Source: three-view drawing plus pictorial views. Frame: mm from the lowest corner of the part. A direction names the side the tool comes from. Give positions to 0.01 mm unless a question says otherwise; leave off trailing zeros. Order: outer loops, then holes, each group sorted by start corner. A loop starts at its lowest first (then second) coordinate and runs counter-clockwise, first axis right, second up. Notation, with made-up numbers: (56.25, 20.25) -> (83.25, 20.25) arc R12 cw to (83.25, 36.25) -> close; hole circle Ø11 at (-9, 13). An arc over 180 degrees is marked (long way). Answer in a Markdown table with one row per item.
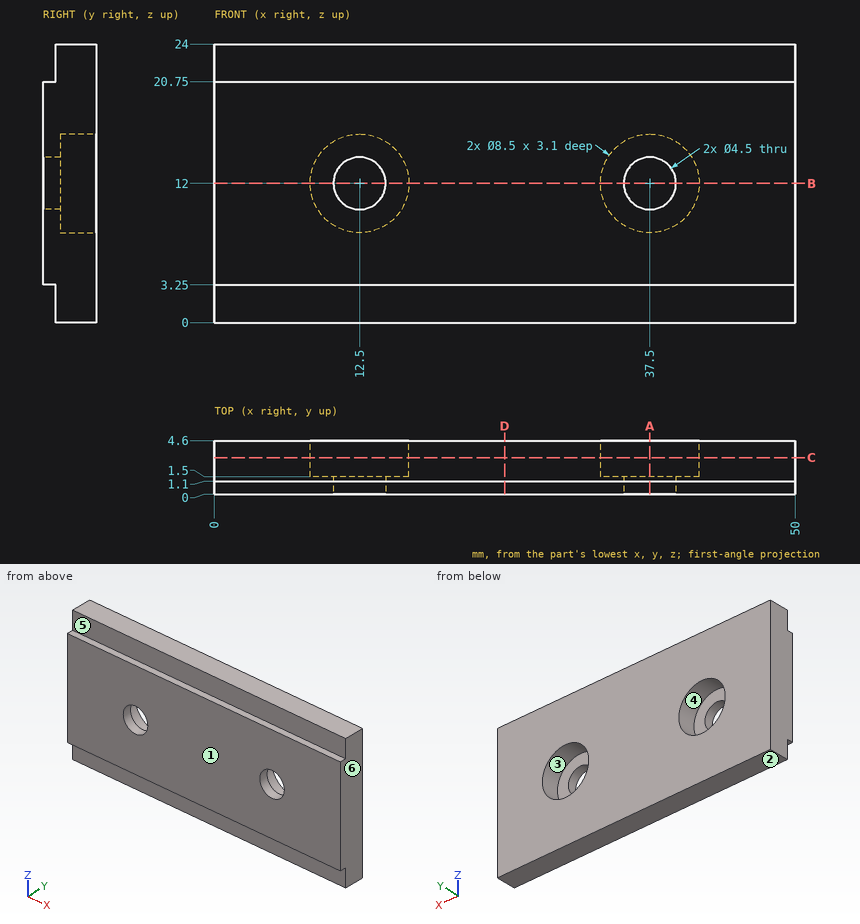
(1) Section query A-A (x = 37.5). Return the cut outline in (y, z), plus the area to 4 significant figures.
A:
| item | result |
|---|---|
| outline | (0, 3.25) -> (1.1, 3.25) -> (1.1, 0) -> (4.6, 0) -> (4.6, 7.75) -> (1.5, 7.75) -> (1.5, 9.75) -> (0, 9.75) -> close; (0, 14.25) -> (1.5, 14.25) -> (1.5, 16.25) -> (4.6, 16.25) -> (4.6, 24) -> (1.1, 24) -> (1.1, 20.75) -> (0, 20.75) -> close |
| area | 70.15 mm^2 |
(2) First-contact query: pin 1 Ø0.6 at (x, y) = (31, 0.5) entering from +Z; pin 2 Ø2.5 at (x, z) = (20, 22.5) entering from -Y; pin 3 Ø7 at (x, z) = (12.5, 12) entering from +Y. Flat tips, straight axial feed; report the tip coordinate or a pass-through.
A:
| item | result |
|---|---|
| pin 1 | stops at z = 20.75 |
| pin 2 | stops at y = 1.1 |
| pin 3 | stops at y = 1.5 |
(3) Section query D-D (x = 25). Return the cut outline in (y, z).
A:
| item | result |
|---|---|
| outline | (0, 3.25) -> (1.1, 3.25) -> (1.1, 0) -> (4.6, 0) -> (4.6, 24) -> (1.1, 24) -> (1.1, 20.75) -> (0, 20.75) -> close |
(4) Pull-direction query (Z, two-part tool) for the marked faces 1, 2 and 3; classes: +Z half, -Z half, draft (parallel to the pull), parting line (faces both ways), or undercut.
A:
| item | result |
|---|---|
| face 1 | draft |
| face 2 | -Z half |
| face 3 | undercut |
(5) Section query B-B (z = 12). Return the cut outline in (x, y), plus the area to 3 significant figures.
A:
| item | result |
|---|---|
| outline | (0, 0) -> (10.25, 0) -> (10.25, 1.5) -> (8.25, 1.5) -> (8.25, 4.6) -> (0, 4.6) -> close; (14.75, 0) -> (35.25, 0) -> (35.25, 1.5) -> (33.25, 1.5) -> (33.25, 4.6) -> (16.75, 4.6) -> (16.75, 1.5) -> (14.75, 1.5) -> close; (39.75, 0) -> (50, 0) -> (50, 4.6) -> (41.75, 4.6) -> (41.75, 1.5) -> (39.75, 1.5) -> close |
| area | 164 mm^2 |
(6) Section query C-C (y = 3.15). Return the cut outline in (x, z), plus the area to 3 significant figures.
A:
| item | result |
|---|---|
| outline | (0, 0) -> (50, 0) -> (50, 24) -> (0, 24) -> close; hole circle Ø8.5 at (12.5, 12); hole circle Ø8.5 at (37.5, 12) |
| area | 1,090 mm^2 |
(7) Access query for the marked faces 4, 5 and 6. Directions: +Z, -Z, +X, -X, +Y, -Y. A direction counts if a zero-diameter tool reaches every point of the face in a straight line with its end or side. Return the directions, or none.
A:
| item | result |
|---|---|
| face 4 | +Y |
| face 5 | +Z, +X, -X, -Y |
| face 6 | +Z, -Z, +X, +Y, -Y |
(8) Ray query, probe 1 along X at (y, z) = (0.45, 12); probe 2 along X at (y, z) = (2.4, 12); probe 3 along Y at (x, z) = (16, 2.75). Return the intervals inside material, ascending.
A:
| item | result |
|---|---|
| probe 1 | x = 0 to 10.25, 14.75 to 35.25, 39.75 to 50 |
| probe 2 | x = 0 to 8.25, 16.75 to 33.25, 41.75 to 50 |
| probe 3 | y = 1.1 to 4.6 |
